Could you check a few things on this model? Use its own coordinates, in mm. Face numbers are marked on the shaded views. Coordinates: 2 decimals unless noted, no trailing zeros. Loops run counter-clockwise (first coordinate to the right, second up) from the corner with the lowest first, then second, coordinate; pieces in that order, holes last.
1) If I drill on line 1 along Z through (x, y) = (-20, -2); line 2 along X through (y, z) = (-68, 94); line 3 along X through (y, z) = (-38.5, 60.5), over which ranges is the centre line in solid material (lowest first)?
2) Thinking about a two-plate mould opening in X: for the marked faces 1, 2 and 3, which applies, released by +X, released by -X, zero draft, split by the parting line, or undercut?
3) Imagine slicing it at C-C on y = -23. Please give me the cut outline in (x, z), plus the area to 3 significant figures.
4) Will these pins go through, and if not, where does the flat tip stop? P1, Ø1.5, axis at y = -59.5, z = 93.5, coming from the -X side; P2, Ø1.5, axis at x = -45.5, y = 53.5, coming from the -Z side; P3, Ø10, axis at y = -19.5, z = 30, coming from the -X side.
5) Imagine slicing it at B-B on y = -55.5. Please give me the cut outline in (x, z), plus the area to 4 significant figures.
6) Imagine slicing it at D-D on x = 64.5. Please give me the cut outline in (y, z).
7) Imagine slicing it at A-A on z = 101. Please give me the cut outline in (x, y), plus the area to 3 significant figures.
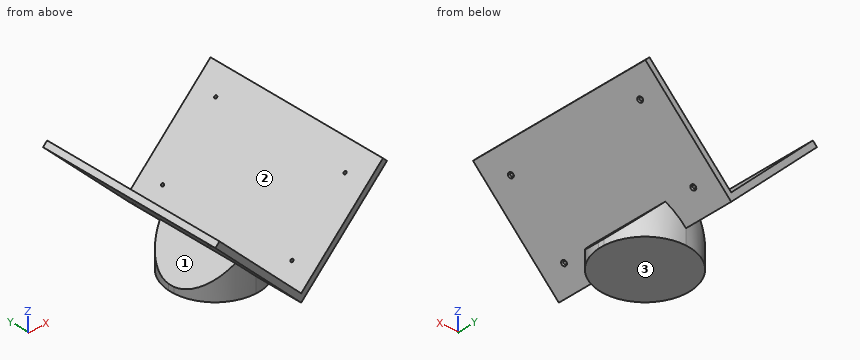
```python
from build123d import *

# Parameters (mm, degrees)
BOSS_EXTRUDE1_START                             = -38.1
BOSS_EXTRUDE1_DEPTH                             = 76.2
BOSS_EXTRUDE1_START_2                           = 20
BOSS_EXTRUDE1_2_DEPTH                           = 29
BOSS_EXTRUDE2_DEPTH                             = 80
CSK_FOR_M2_FLAT_HEAD_MACHINE_SCREW1_D           = 2.4
CSK_FOR_M2_FLAT_HEAD_MACHINE_SCREW1_CSINK_D     = 4.4
CSK_FOR_M2_FLAT_HEAD_MACHINE_SCREW1_CSINK_ANGLE = 90


with BuildPart() as part:
    # Boss-Extrude1: read off the stored shape, not the designer's step
    # Boss-Extrude1 outline → Boss-Extrude1 (new body)
    with BuildSketch(Plane(origin=(0, 0, 0), x_dir=(1, 0, 0), z_dir=(0, 1, 0)).offset(BOSS_EXTRUDE1_START)):
        Polygon((-15, -48.011182565), (0, -33.011182565), (15, -48.011182565), (38.011182565, -25), (38.011182565, -20), (-38.011182565, -20), (-38.011182565, -25), align=None)
    extrude(amount=BOSS_EXTRUDE1_DEPTH)

    # Boss-Extrude1 2 outline → Boss-Extrude1 2 (cut)
    with BuildSketch(Plane.XY.offset(BOSS_EXTRUDE1_START_2)):
        with BuildLine():
            ThreePointArc((0, 38.1), (26.005287924, 27.844837942), (38.011182565, 2.6))
            Line((38.011182565, 2.6), (38.011182565, 38.1))
            Line((38.011182565, 38.1), (0, 38.1))
        make_face()
        with BuildLine():
            ThreePointArc((-38.011182565, 2.6), (-26.005287924, 27.844837942), (0, 38.1))
            Line((0, 38.1), (-38.011182565, 38.1))
            Line((-38.011182565, 38.1), (-38.011182565, 2.6))
        make_face()
        with BuildLine():
            Line((38.011182565, -38.1), (38.011182565, -2.6))
            ThreePointArc((38.011182565, -2.6), (26.005287924, -27.844837942), (0, -38.1))
            Line((0, -38.1), (38.011182565, -38.1))
        make_face()
        with BuildLine():
            Line((-38.011182565, -38.1), (0, -38.1))
            ThreePointArc((0, -38.1), (-26.005287924, -27.844837942), (-38.011182565, -2.6))
            Line((-38.011182565, -2.6), (-38.011182565, -38.1))
        make_face()
    extrude(amount=BOSS_EXTRUDE1_2_DEPTH, mode=Mode.SUBTRACT)

    # Sketch1<3> → Boss-Extrude2 (add, symmetric)
    with BuildSketch(Plane(origin=(0, 0, 0), x_dir=(1, 0, 0), z_dir=(0, 1, 0))):
        Polygon((0, -33.011182565), (15, -48.011182565), (74.246212025, -107.25739459), (70.710678119, -110.792928496), (0, -40.082250377), (-70.710678119, -110.792928496), (-74.246212025, -107.25739459), (-15, -48.011182565), align=None)
    extrude(amount=BOSS_EXTRUDE2_DEPTH, both=True)

    # CSK for M2 Flat Head Machine Screw1 (through all)
    with Locations(Plane(origin=(16.505591283, 0, 16.505591283), x_dir=(-0.7071067811865441, 0, 0.7071067811865509), z_dir=(-0.7071067811865509, 0, -0.7071067811865441))):
        with Locations((108.342431047, 60), (43.342431047, 60), (43.342431047, -60), (108.342431047, -60)):
            csk_for_m2_flat_head_machine_screw1 = CounterSinkHole(CSK_FOR_M2_FLAT_HEAD_MACHINE_SCREW1_D / 2, CSK_FOR_M2_FLAT_HEAD_MACHINE_SCREW1_CSINK_D / 2, counter_sink_angle=CSK_FOR_M2_FLAT_HEAD_MACHINE_SCREW1_CSINK_ANGLE)

    # Mirror1: CSK for M2 Flat Head Machine Screw1 across plane
    add(csk_for_m2_flat_head_machine_screw1.mirror(Plane(origin=(0, 0, 0), x_dir=(0, 0, 1), z_dir=(1, 0, 0))), mode=Mode.SUBTRACT)


solid = part.part
```
Filled in:
1. line 1: z = 20 to 43.01, 53.01 to 60.08
1. line 2: x = -60.99 to -53.92, 53.92 to 60.99
1. line 3: x = -27.49 to -20.42, 20.42 to 27.49
2. face 1: released by -X
2. face 2: undercut
2. face 3: zero draft
3. outline: (-74.25, 107.26) - (-15, 48.01) - (-30.37, 32.64) - (-30.37, 20) - (30.37, 20) - (30.37, 32.64) - (15, 48.01) - (74.25, 107.26) - (70.71, 110.79) - (0, 40.08) - (-70.71, 110.79) - close
3. area: 2,270 mm2
4. P1: stops at x = -59.35
4. P2: stops at z = 77.76
4. P3: stops at x = -35.05
5. outline: (-74.25, 107.26) - (0, 33.01) - (74.25, 107.26) - (70.71, 110.79) - (0, 40.08) - (-70.71, 110.79) - close
5. area: 1,025 mm2
6. outline: (-80, 97.51) - (80, 97.51) - (80, 104.58) - (-80, 104.58) - close
7. outline: (-67.99, -80) - (-60.92, -80) - (-60.92, 80) - (-67.99, 80) - close; (60.92, -80) - (67.99, -80) - (67.99, 80) - (60.92, 80) - close
7. area: 2,260 mm2
